from build123d import *

# Parameters (mm, degrees)
SKETCH1_W                 = 46
SKETCH1_H                 = 26
BOSS_EXTRUDE1_DEPTH       = 27.6
SKETCH2_W                 = 66
SKETCH2_H                 = 26
BOSS_EXTRUDE2_DEPTH       = 10.1
SKETCH3_W                 = 40
SKETCH3_H                 = 20
CUT_EXTRUDE2_DEPTH        = 25.5
F_1_5MM_DOWEL_HOLE2_D     = 1.5
F_1_5MM_DOWEL_HOLE2_DEPTH = 9
F_1_5MM_DOWEL_HOLE2_TIP   = 0.450645464
SKETCH8_W                 = 40
SKETCH8_H                 = 20
CUT_EXTRUDE6_DEPTH        = 3
SKETCH7_W                 = 16
SKETCH7_H                 = 15
CUT_EXTRUDE8_DEPTH        = 3
SKETCH9_R                 = 10.9
CUT_EXTRUDE9_DEPTH        = 7
SKETCH10_W                = 44
SKETCH10_H                = 20
CUT_EXTRUDE10_DEPTH       = 28.5
SKETCH11_W                = 26
SKETCH11_H                = 27.6
BOSS_EXTRUDE3_DEPTH       = 10
F_2_5MM_DOWEL_HOLE1_D     = 2.5
F_2_5MM_DOWEL_HOLE1_DEPTH = 26
F_2_5MM_DOWEL_HOLE1_TIP   = 0.751075774
F_2_5MM_DOWEL_HOLE2_D     = 2.5
F_2_5MM_DOWEL_HOLE2_DEPTH = 9
F_2_5MM_DOWEL_HOLE2_TIP   = 0.751075774


with BuildPart() as part:
    # Sketch1 → Boss-Extrude1 (new body)
    with BuildSketch(Plane(origin=(0, 0, 0), x_dir=(1, 0, 0), z_dir=(0, 1, 0))):
        with Locations((23, 13)):
            Rectangle(SKETCH1_W, SKETCH1_H)
    extrude(amount=BOSS_EXTRUDE1_DEPTH)

    # Sketch2 → Boss-Extrude2 (add)
    with BuildSketch(Plane(origin=(0, 27.6, 0), x_dir=(1, 0, 0), z_dir=(0, 1, 0))):
        with Locations((23, 13)):
            Rectangle(SKETCH2_W, SKETCH2_H)
    extrude(amount=BOSS_EXTRUDE2_DEPTH)

    # Sketch3 → Cut-Extrude2 (cut)
    with BuildSketch(Plane(origin=(0, 37.7, 0), x_dir=(1, 0, 0), z_dir=(0, 1, 0))):
        with Locations((23, 13)):
            Rectangle(SKETCH3_W, SKETCH3_H)
    extrude(amount=-CUT_EXTRUDE2_DEPTH, mode=Mode.SUBTRACT)

    # Ø1.5mm Dowel Hole2
    with Locations(Plane(origin=(-1.9, 37.7, -18), x_dir=(0, 0, 1), z_dir=(0, 1, 0))):
        with Locations((0, 0), (10, 0), (10, 49.7), (0, 49.8)):
            Hole(F_1_5MM_DOWEL_HOLE2_D / 2, depth=F_1_5MM_DOWEL_HOLE2_DEPTH)
            with Locations((0, 0, -(F_1_5MM_DOWEL_HOLE2_DEPTH + F_1_5MM_DOWEL_HOLE2_TIP / 2))):  # 118° drill point
                Cone(0, F_1_5MM_DOWEL_HOLE2_D / 2, F_1_5MM_DOWEL_HOLE2_TIP, mode=Mode.SUBTRACT)

    # Sketch8 → Cut-Extrude6 (cut)
    with BuildSketch(Plane(origin=(0, 12.2, 0), x_dir=(1, 0, 0), z_dir=(0, 1, 0))):
        with Locations((23, 13)):
            Rectangle(SKETCH8_W, SKETCH8_H)
    extrude(amount=-CUT_EXTRUDE6_DEPTH, mode=Mode.SUBTRACT)

    # Sketch7 → Cut-Extrude8 (cut)
    with BuildSketch(Plane.ZY):
        with Locations((-13, 19.5)):
            Rectangle(SKETCH7_W, SKETCH7_H)
    extrude(amount=-CUT_EXTRUDE8_DEPTH, mode=Mode.SUBTRACT)

    # Sketch9 → Cut-Extrude9 (cut)
    with BuildSketch(Plane(origin=(0, 0, 0), x_dir=(-1, 0, 0), z_dir=(0, -1, 0))):
        with Locations(Location((-13.05, 13, 0), (0, 0, 90))):
            Circle(SKETCH9_R)
    extrude(amount=-CUT_EXTRUDE9_DEPTH, mode=Mode.SUBTRACT)

    # Sketch10 → Cut-Extrude10 (cut)
    with BuildSketch(Plane(origin=(0, 37.7, 0), x_dir=(1, 0, 0), z_dir=(0, 1, 0))):
        with Locations((23, 13)):
            Rectangle(SKETCH10_W, SKETCH10_H)
    extrude(amount=-CUT_EXTRUDE10_DEPTH, mode=Mode.SUBTRACT)

    # Sketch11 → Boss-Extrude3 (add)
    with BuildSketch(Plane(origin=(46, 0, 0), x_dir=(0, 0, -1), z_dir=(1, 0, 0))):
        with Locations((13, 13.8)):
            Rectangle(SKETCH11_W, SKETCH11_H)
    extrude(amount=BOSS_EXTRUDE3_DEPTH)

    # Ø2.5mm Dowel Hole1
    with Locations(Plane(origin=(51, 18.4, 0), x_dir=(1, 0, 0), z_dir=(0, 0, 1))):
        with Locations((0, 0), (0, -9.2)):
            Hole(F_2_5MM_DOWEL_HOLE1_D / 2, depth=F_2_5MM_DOWEL_HOLE1_DEPTH)
            with Locations((0, 0, -(F_2_5MM_DOWEL_HOLE1_DEPTH + F_2_5MM_DOWEL_HOLE1_TIP / 2))):  # 118° drill point
                Cone(0, F_2_5MM_DOWEL_HOLE1_D / 2, F_2_5MM_DOWEL_HOLE1_TIP, mode=Mode.SUBTRACT)

    # Ø2.5mm Dowel Hole2
    with Locations(Plane.XZ):
        with Locations((51, -13)):
            Hole(F_2_5MM_DOWEL_HOLE2_D / 2, depth=F_2_5MM_DOWEL_HOLE2_DEPTH)
            with Locations((0, 0, -(F_2_5MM_DOWEL_HOLE2_DEPTH + F_2_5MM_DOWEL_HOLE2_TIP / 2))):  # 118° drill point
                Cone(0, F_2_5MM_DOWEL_HOLE2_D / 2, F_2_5MM_DOWEL_HOLE2_TIP, mode=Mode.SUBTRACT)


solid = part.part
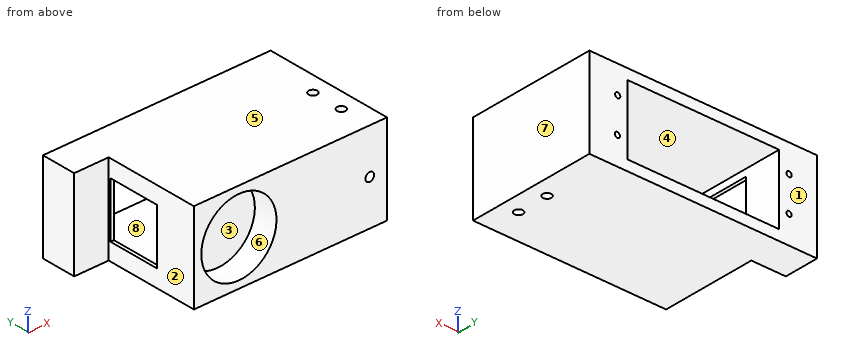
Verification items for the finished model (mm, model axes). Face numbers are marked on the shaded views. A direction names the side the tool comes from. Give positions to 0.01 mm unless a question says otherwise; leave off trailing zeros. Loops run counter-clockwise (first coordinate to the right, second up) from the corner with the lowest first, then second, coordinate; pieces in that order, holes last.
1) Thickness scan on line 1 along Z through (x, y) = (-1.9, 32.75); line 2 along Y through (x, z) = (51, -11.5); line 3 along X through (y, z) = (3, -13). Record the ranges inside material, lowest first.
2) Sectioned sample at B-B, the plane z = -6.5. Enter the section's corners in (x, y).
3) Draft check along X on the marked faces 5, 6, 7 and 8. Enter one of: pulls with the +X half, pulls with the -X half, needs draft (parallel to the pull), parting line crosses it, or undercut.
4) Sectioned sample at C-C, the plane y = 35. Enter the section's corners in (x, z), then the cut area to 3 significant figures.
5) Sectioned sample at A-A, the plane y = 18.4. Enter the section's corners in (x, z), then the cut area to 3 significant figures.
6) Sectioned sample at D-D, the plane x = 13.05. Enter the section's corners in (y, z), then the cut area to 3 significant figures.
7) Depth check by flat-ended pin: pin 1 Ø10 at (x, z) = (16, -10.5) entering from +Y; pin 2 Ø3 at (y, z) = (13, -23) entering from -X; pin 3 Ø1.2 at (x, z) = (-1.9, -8) entering from +Y. Enter the tip coordinate at first touch or a pass-through.
8) Set-up check for the marked faces 1, 2, 3 and 4: record each of +Z, -Z, +X, -X, +Y, -Y from which the full face is reachable in a straight line by a thin tool's end or side.
Answers:
1. line 1: z = -26 to -18.75, -17.25 to -8.75, -7.25 to 0
1. line 2: y = 0 to 7.95, 10.45 to 17.15, 19.65 to 37.7
1. line 3: x = 0 to 2.15, 23.95 to 49.75, 52.25 to 56
2. outline: (-10, 27.6) - (0, 27.6) - (0, 27) - (1, 27) - (1, 37.7) - (-10, 37.7) - close; (0, 0) - (4.3, 0) - (4.3, 7) - (21.8, 7) - (21.8, 0) - (56, 0) - (56, 37.7) - (45, 37.7) - (45, 9.2) - (1, 9.2) - (1, 12) - (0, 12) - close; hole circle Ø2.5 at (51, 9.2); hole circle Ø2.5 at (51, 18.4)
3. face 5: needs draft
3. face 6: undercut
3. face 7: pulls with the +X half
3. face 8: undercut
4. outline: (-10, -26) - (56, -26) - (56, 0) - (-10, 0) - close; hole circle Ø1.5 at (-1.9, -18); hole circle Ø1.5 at (-1.9, -8); hole (1, -23) - (45, -23) - (45, -3) - (1, -3) - close; hole circle Ø1.5 at (47.8, -8); hole circle Ø1.5 at (47.9, -18)
4. area: 829 mm2
5. outline: (0, -26) - (49.75, -26) - (49.75, 0) - (0, 0) - (0, -5) - (1, -5) - (1, -3) - (45, -3) - (45, -23) - (1, -23) - (1, -21) - (0, -21) - close; (52.25, -26) - (56, -26) - (56, 0) - (52.25, 0) - close
5. area: 495 mm2
6. outline: (0, -26) - (37.7, -26) - (37.7, -23) - (9.2, -23) - (9.2, -3) - (37.7, -3) - (37.7, 0) - (0, 0) - (0, -2.1) - (7, -2.1) - (7, -23.9) - (0, -23.9) - close
6. area: 258 mm2
7. pin 1: stops at y = 9.2
7. pin 2: stops at x = 0
7. pin 3: stops at y = 28.61
8. face 1: +Z, -Z, +X, -X, +Y
8. face 2: +Z, -Z, -X, -Y
8. face 3: -Y
8. face 4: +Y
